Can you work these out from the model? Positions are in its coordinate system, mm. A direction names the side the tool comes from. Give positions to 0.01 mm unless a question says otherwise; leave off trailing zeros. Loops run counter-clockwise (first coordinate to the right, second up) from the corner with the lowest first, then second, coordinate; pieces in that order, holes last. Notation, with made-up numbers: (26.5, -6) - (71.5, -6) arc R10 ccw to (71.5, -1) - close; hole circle Ø11 at (36.5, -27.75). An arc over 180 degrees is marked (long way). Use a Markdown table: item, result. Add a question column.
```python
from build123d import *

# Parameters (mm, degrees)
CUT_EXTRUDE1_DEPTH      = 69.067346778
CUT_EXTRUDE1_DEPTH_BACK = 69.067346778
SKETCH3_R               = 7.366


with BuildPart() as part:
    # Sketch2 → Revolve1 (revolve)
    with BuildSketch(Plane(origin=(0, 0, 0), x_dir=(1, 0, 0), z_dir=(0, 1, 0))):
        Polygon((-5.831340186, 11.938), (4.767118223, 11.938), (4.767118223, 10.563948577), (18.927664498, 10.563948577), (18.927664498, 12.948727397), (23.441288756, 12.948727397), (23.441288756, 14.231007016), (30.170692197, 14.231007016), (30.170692197, 12.013405261), (44.121894451, 12.013405261), (44.121894451, 14.231007016), (56.23516923, 14.231007016), (56.23516923, 9.700025704), (59.192659814, 9.700025704), (59.192659814, 0), (-5.831340186, 0), align=None)
    revolve(axis=Axis((59.192659814, 0, 0), (-1, 0, 0)))

    # Sketch3 → Cut-Extrude1 (cut, two sides: drawn at the far end of the back side and taken through both)
    with BuildSketch(Plane(origin=(59.192659814, 0, 0), x_dir=(0, 0, -1), z_dir=(1, 0, 0)).offset(-CUT_EXTRUDE1_DEPTH_BACK)):
        Circle(SKETCH3_R)
    extrude(amount=CUT_EXTRUDE1_DEPTH + CUT_EXTRUDE1_DEPTH_BACK, mode=Mode.SUBTRACT)


solid = part.part
```
1. Suppose I cut it at C-C (x = 15). List the corners of the cut face in (y, z) for me, and give its area (3 significant figures).
2. If we mould it in two halves opening along X, with no side actions, what happens to faces 5 (the face through (30.171, 7, 10)), 6 (the face through (-5.831, 8, 0)), 7 (the face through (18.928, 0, -11)), 8 (the face through (26.853, -4.275, -13.574))? For each: released by +X, released by -X, zero draft, split by the parting line, or undercut.
3. On a 3-axis mill with a long thin cutter (end or side, diameter ignored), from which of +Z, -Z, +X, -X, +Y, -Y can I reach the whole of each face in a straight line? I mean faces 1 (the face through (-0.458, 11.654, 2.588)), 2 (the face through (56.235, 9.3, 3.4)), 3 (the face through (59.193, -7.23, -2.11)), 4 (the face through (37.24, 11.73, 2.6)). Say none if no direction works.
4. Please list where these lines run through material, in increasing order: line 1 along X through (y, z) = (-9.5, -4.75); line 2 along Y through (x, z) = (18, 0). Write a range as [from, to].
5. Will these pins go through, and if not, where does the flat tip stop? P1, Ø12, axis at x = 14.5, z = 11.5, coming from the +Y side; P2, Ø10, axis at x = 25.5, z = -8, coming from the +Y side; P3, Ø12, axis at y = -3.5, z = -1.5, coming from the +X side; P4, Ø1.5, axis at x = 39, z = 6.5, coming from the -Y side.
6. Suppose I cut it at D-D (z = -8). List the corners of the cut face in (x, y) for me.
Results below:
| question | item | result |
|---|---|---|
| 1 | outline | circle Ø21.13 at (0, 0); hole circle Ø14.73 at (0, 0) |
| 1 | area | 180 mm² |
| 2 | face 5 | undercut |
| 2 | face 6 | released by -X |
| 2 | face 7 | undercut |
| 2 | face 8 | zero draft |
| 3 | face 1 | -X |
| 3 | face 2 | +X |
| 3 | face 3 | +Z, -Z, +X, +Y, -Y |
| 3 | face 4 | none |
| 4 | line 1 | [-5.83, 4.77], [18.93, 56.24] |
| 4 | line 2 | [-10.56, -7.37], [7.37, 10.56] |
| 5 | P1 | y = 10.59 |
| 5 | P2 | y = 13.91 |
| 5 | P3 | x = 59.19 |
| 5 | P4 | y = -10.55 |
| 6 | outline | (-5.83, -8.86) - (4.77, -8.86) - (4.77, -6.9) - (18.93, -6.9) - (18.93, -10.18) - (23.44, -10.18) - (23.44, -11.77) - (30.17, -11.77) - (30.17, -8.96) - (44.12, -8.96) - (44.12, -11.77) - (56.24, -11.77) - (56.24, -5.49) - (59.19, -5.49) - (59.19, 5.49) - (56.24, 5.49) - (56.24, 11.77) - (44.12, 11.77) - (44.12, 8.96) - (30.17, 8.96) - (30.17, 11.77) - (23.44, 11.77) - (23.44, 10.18) - (18.93, 10.18) - (18.93, 6.9) - (4.77, 6.9) - (4.77, 8.86) - (-5.83, 8.86) - close |
